```python
from build123d import *

# Parameters (mm, degrees)
SKETCH1_R           = 2.1
BOSS_EXTRUDE1_DEPTH = 100


with BuildPart() as part:
    # Sketch1 → Boss-Extrude1 (new body)
    with BuildSketch(Plane(origin=(0, 0, 0), x_dir=(0, 0, -1), z_dir=(1, 0, 0))):
        with BuildLine():
            Line((-10, 7), (-10, -7))
            Line((-10, -7), (-8, -7))
            Line((-8, -7), (-8, -4))
            Line((-8, -4), (-7.060660172, -4))
            Line((-7.060660172, -4), (-4, -7.060660172))
            Line((-4, -7.060660172), (-4, -12.939339828))
            Line((-4, -12.939339828), (-7.060660172, -16))
            Line((-7.060660172, -16), (-8, -16))
            Line((-8, -16), (-8, -13))
            Line((-8, -13), (-10, -13))
            Line((-10, -13), (-10, -19))
            ThreePointArc((-10, -19), (-9.948683298, -19.316227766), (-9.8, -19.6))
            Line((-9.8, -19.6), (-3, -19.6))
            Line((-3, -19.6), (-3, -18))
            Line((-3, -18), (-6, -18))
            Line((-6, -18), (-6, -17.060660172))
            Line((-6, -17.060660172), (-2.939339828, -14))
            Line((-2.939339828, -14), (2.939339828, -14))
            Line((2.939339828, -14), (6, -17.060660172))
            Line((6, -17.060660172), (6, -18))
            Line((6, -18), (3, -18))
            Line((3, -18), (3, -19.6))
            Line((3, -19.6), (9.8, -19.6))
            ThreePointArc((9.8, -19.6), (9.948683298, -19.316227766), (10, -19))
            Line((10, -19), (10, -13))
            Line((10, -13), (8, -13))
            Line((8, -13), (8, -16))
            Line((8, -16), (7.060660172, -16))
            Line((7.060660172, -16), (4, -12.939339828))
            Line((4, -12.939339828), (4, -7.060660172))
            Line((4, -7.060660172), (7.060660172, -4))
            Line((7.060660172, -4), (8, -4))
            Line((8, -4), (8, -7))
            Line((8, -7), (10, -7))
            Line((10, -7), (10, 7))
            Line((10, 7), (8, 7))
            Line((8, 7), (8, 4))
            Line((8, 4), (7.060660172, 4))
            Line((7.060660172, 4), (4, 7.060660172))
            Line((4, 7.060660172), (4, 12.939339828))
            Line((4, 12.939339828), (7.060660172, 16))
            Line((7.060660172, 16), (8, 16))
            Line((8, 16), (8, 13))
            Line((8, 13), (10, 13))
            Line((10, 13), (10, 19))
            ThreePointArc((10, 19), (9.948683298, 19.316227766), (9.8, 19.6))
            Line((9.8, 19.6), (3, 19.6))
            Line((3, 19.6), (3, 18))
            Line((3, 18), (6, 18))
            Line((6, 18), (6, 17.060660172))
            Line((6, 17.060660172), (2.939339828, 14))
            Line((2.939339828, 14), (-2.939339828, 14))
            Line((-2.939339828, 14), (-6, 17.060660172))
            Line((-6, 17.060660172), (-6, 18))
            Line((-6, 18), (-3, 18))
            Line((-3, 18), (-3, 19.6))
            Line((-3, 19.6), (-9.8, 19.6))
            ThreePointArc((-9.8, 19.6), (-9.948683298, 19.316227766), (-10, 19))
            Line((-10, 19), (-10, 13))
            Line((-10, 13), (-8, 13))
            Line((-8, 13), (-8, 16))
            Line((-8, 16), (-7.060660172, 16))
            Line((-7.060660172, 16), (-4, 12.939339828))
            Line((-4, 12.939339828), (-4, 7.060660172))
            Line((-4, 7.060660172), (-7.060660172, 4))
            Line((-7.060660172, 4), (-8, 4))
            Line((-8, 4), (-8, 7))
            Line((-8, 7), (-10, 7))
        make_face()
        with Locations((0, 10)):
            Circle(SKETCH1_R, mode=Mode.SUBTRACT)
        with Locations((0, -10)):
            Circle(SKETCH1_R, mode=Mode.SUBTRACT)
        with BuildLine():
            Line((-8, 1.7), (-8, -1.7))
            ThreePointArc((-8, -1.7), (-7.912132034, -1.912132034), (-7.7, -2))
            Line((-7.7, -2), (-7.063603897, -2))
            ThreePointArc((-7.063603897, -2), (-6.948798867, -2.02283614), (-6.851471863, -2.087867966))
            Line((-6.851471863, -2.087867966), (-2.939339828, -6))
            Line((-2.939339828, -6), (2.939339828, -6))
            Line((2.939339828, -6), (6.851471863, -2.087867966))
            ThreePointArc((6.851471863, -2.087867966), (6.948798867, -2.02283614), (7.063603897, -2))
            Line((7.063603897, -2), (7.7, -2))
            ThreePointArc((7.7, -2), (7.912132034, -1.912132034), (8, -1.7))
            Line((8, -1.7), (8, 1.7))
            ThreePointArc((8, 1.7), (7.912132034, 1.912132034), (7.7, 2))
            Line((7.7, 2), (7.063603897, 2))
            ThreePointArc((7.063603897, 2), (6.948798867, 2.02283614), (6.851471863, 2.087867966))
            Line((6.851471863, 2.087867966), (2.939339828, 6))
            Line((2.939339828, 6), (-2.939339828, 6))
            Line((-2.939339828, 6), (-6.851471863, 2.087867966))
            ThreePointArc((-6.851471863, 2.087867966), (-6.948798867, 2.02283614), (-7.063603897, 2))
            Line((-7.063603897, 2), (-7.7, 2))
            ThreePointArc((-7.7, 2), (-7.912132034, 1.912132034), (-8, 1.7))
        make_face(mode=Mode.SUBTRACT)
    extrude(amount=BOSS_EXTRUDE1_DEPTH)


solid = part.part
```
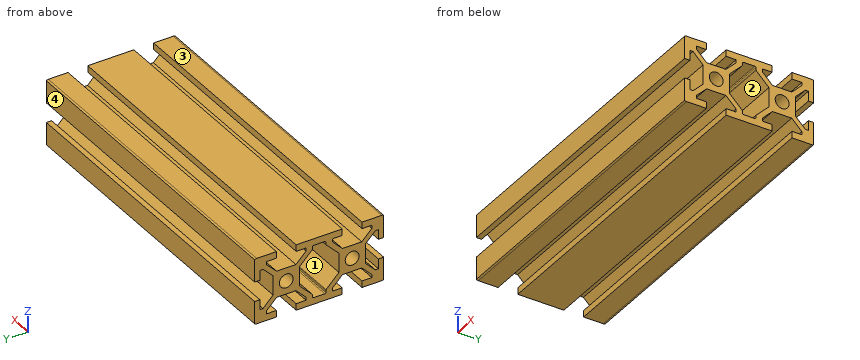
Work out the finished part from the listing and answer in its coordinate system (mm). Face numbers are marked on the shaded views. Coordinates: 2 decimals unless noted, no trailing zeros. Write each loop counter-clockwise with the first axis right and the second up, starting at its lowest first coordinate (ties: lowest second). Pieces come first, ordered by that corner, then holes.
Q1. Each of these flat-tipped pins is pushed along its axis until it touches: pin 1 Ø3 at (x, y) = (41, -10) entering from +Z; pin 2 Ø1.8 at (x, y) = (49.5, -9.5) entering from -Z; pin 3 Ø4.5 at (x, z) = (32, 0.5) entering from +Y. Where does it stop, or does it pass through?
Q2. Find the intervals of material crossed by line 1 (Y direction, x = 49, z = 0); line 2 (Y direction, x = 7.5, z = 8.25); line 3 (Y direction, x = 9.5, z = 2.75), in increasing order.
Q3. A cutting plane is placed at B-B, the plane y = 10. Give the vertices of the cut face in (x, z), then the cut area to 3 significant figures.
Q4. A cutting plane is placed at A-A, the plane z = 0. Give the vertices of the cut face in (x, y), then the cut area to 3 significant figures.
Q5. A cutting plane is placed at C-C, the plane x = 32. State how many separate pieces and enclosed holes the cut face has, then the cut area to 3 significant figures.
Q6. Determine the mould class of the marked faces 1, 2, 3 and 4 for opening direction Y: released by +Y, released by -Y, zero draft, split by the parting line, or undercut.
Findings below:
1. pin 1: stops at z = 4
1. pin 2: stops at z = -4
1. pin 3: stops at y = 14
2. line 1: y = -14 to -12.1, -7.9 to -6, 6 to 7.9, 12.1 to 14
2. line 2: y = -19.6 to -13, -7 to 7, 13 to 19.6
2. line 3: y = -14 to -6, 6 to 14
3. outline: (0, -4) - (100, -4) - (100, -2.1) - (0, -2.1) - close; (0, 2.1) - (100, 2.1) - (100, 4) - (0, 4) - close
3. area: 380 mm2
4. outline: (0, -14) - (100, -14) - (100, -12.1) - (0, -12.1) - close; (0, -7.9) - (100, -7.9) - (100, -6) - (0, -6) - close; (0, 6) - (100, 6) - (100, 7.9) - (0, 7.9) - close; (0, 12.1) - (100, 12.1) - (100, 14) - (0, 14) - close
4. area: 760 mm2
5. separate pieces: 1
5. enclosed holes: 3
5. area: 314 mm2
6. face 1: undercut
6. face 2: undercut
6. face 3: zero draft
6. face 4: released by +Y
